For this review, take the finished solid that the model builds, in its own axes (mm). Face numbers are marked on the shaded views. A direction names the side the tool comes from. Round coordinates to 2 decimals unless told otherwise and drop trailing zeros. Loops run counter-clockwise (first coordinate to the right, second up) from the corner with the lowest first, then second, coordinate; pieces in that order, holes last.
1. Tool access review of the marked faces 1, 2 and 3: name each direction out of +Z, -Z, +X, -X, +Y, -Y from which nothing blocks a thin tool from reaching the whole face with its end or side.
2. Draft analysis for pull direction X (two halves, no side actions). For the marked faces 4, 5 and 6, state which applies: released by +X, released by -X, zero draft, split by the parting line, or undercut.
3. Clearance check with flat-ended pins moving along their axes: pin 1 Ø0.8 at (y, z) = (-4, 14.5) entering from -X (3 decimals); pin 2 Ø2 at (y, z) = (-2, 10) entering from +X (3 decimals); pin 3 Ø1.4 at (x, y) = (-7.5, -3.5) entering from -Z; pin 4 Ø4 at (x, y) = (-2.5, -3.5) entering from +Z. State where each tip first meets the part, or that it passes through.
4. Consider section A-A on z = 7.5. State the section outline as (x, y) points (3 decimals), then the cut area to 3 significant figures.
5. Consider section D-D on y = -2.5. State how many separate pieces and enclosed holes the cut face has, then the cut area to 3 significant figures.
6. To check wall thickness, follow line 1 along Y through (x, z) = (0, 8.5); line 2 along Z through (x, y) = (-6.5, -1.75); line 3 along Z through (x, y) = (3.5, -2.75). State the ranges of each line that lie inside material, in increasing order.
7. Consider section C-C on z = 11.25. State the section outline as (x, y) points (3 decimals).
from build123d import *

# Parameters (mm, degrees)
SKIZZE1_W                         = 6.675
SKIZZE1_H                         = 4.27
AUFSATZ_LINEAR_AUSTRAGEN1_DEPTH   = 10.4
SKIZZE1_3_W                       = 6.675
SKIZZE1_3_H                       = 1.68
AUFSATZ_LINEAR_AUSTRAGEN2_DEPTH   = 15.35
LINEAR_AUSTRAGEN_D_NN1_START      = 4.75
LINEAR_AUSTRAGEN_D_NN1_DEPTH      = 2
SKIZZE3_W                         = 0.5
SKIZZE3_H                         = 1.6
AUFSATZ_LINEAR_AUSTRAGEN3_DEPTH   = 4.8
SKIZZE4_W                         = 7.337223246
SKIZZE4_H                         = 4.95
SCHNITT_LINEAR_AUSTRAGEN1_DEPTH   = 8.85
AUFSATZ_LINEAR_AUSTRAGEN4_REACH   = 21.408
AUFSATZ_LINEAR_START              = 0.5
SKIZZE5_W                         = 5.4
SKIZZE5_H                         = 2
AUFSATZ_LINEAR_START_2            = -0.9
SKIZZE6_W                         = 0.55
SKIZZE6_H                         = 0.3
AUFSATZ_LINEAR_AUSTRAGEN5_DEPTH   = 3.5
AUFSATZ_LINEAR_AUSTRAGEN5_2_DEPTH = 3.5
SKIZZE6_3_W                       = 0.55
SKIZZE6_3_H                       = 0.2
AUFSATZ_LINEAR_AUSTRAGEN6_DEPTH   = 0.3
VERRUNDUNG1_R                     = 0.2
VERRUNDUNG2_R                     = 0.5
VERRUNDUNG3_R                     = 0.3
VERRUNDUNG4_R                     = 0.7
AUFSATZ_LINEAR_START_3            = -6.675
SKIZZE7_W                         = 2.54
SKIZZE7_H                         = 3.27
AUFSATZ_LINEAR_AUSTRAGEN7_DEPTH   = 0.25
VERRUNDUNG6_R                     = 0.5
VERRUNDUNG7_R                     = 0.5
LINEAR_AUSTRAGEN_D_NN2_DEPTH      = 0.7
VERRUNDUNG5_R                     = 0.7


with BuildPart() as part:
    # Skizze1 → Aufsatz-Linear austragen1 (new body)
    with BuildSketch(Plane.XY):
        with Locations((-3.3375, -3.815)):
            Rectangle(SKIZZE1_W, SKIZZE1_H)
    extrude(amount=AUFSATZ_LINEAR_AUSTRAGEN1_DEPTH)

    # Skizze1<3> → Aufsatz-Linear austragen2 (add)
    with BuildSketch(Plane.XY):
        with Locations((-3.3375, -0.84)):
            Rectangle(SKIZZE1_3_W, SKIZZE1_3_H)
    extrude(amount=AUFSATZ_LINEAR_AUSTRAGEN2_DEPTH)

    # Skizze2 → Linear-Austragen-Dünn1 (add)
    with BuildSketch(Plane.XY.offset(LINEAR_AUSTRAGEN_D_NN1_START)):
        with BuildLine():
            Line((0, -2.95), (-8.75, -2.95))
            ThreePointArc((-8.75, -2.95), (-9.13890873, -3.11109127), (-9.3, -3.5))
            Line((-9.3, -3.5), (-9.3, -4.7))
            Line((-9.3, -4.7), (-8.8, -4.7))
            Line((-8.8, -4.7), (-8.8, -3.5))
            ThreePointArc((-8.8, -3.5), (-8.785355339, -3.464644661), (-8.75, -3.45))
            Line((-8.75, -3.45), (0, -3.45))
            Line((0, -3.45), (0, -2.95))
        make_face()
    extrude(amount=LINEAR_AUSTRAGEN_D_NN1_DEPTH)

    # Skizze3 → Aufsatz-Linear austragen3 (add)
    with BuildSketch(Plane(origin=(0, 0, 0), x_dir=(1, 0, 0), z_dir=(0, 1, 0))):
        with Locations((-6.425, -14.55)):
            Rectangle(SKIZZE3_W, SKIZZE3_H)
    extrude(amount=-AUFSATZ_LINEAR_AUSTRAGEN3_DEPTH)

    # Skizze4 → Schnitt-Linear austragen1 (cut)
    with BuildSketch(Plane.XY):
        with Locations((-2.511388377, -2.975)):
            Rectangle(SKIZZE4_W, SKIZZE4_H)
    extrude(amount=SCHNITT_LINEAR_AUSTRAGEN1_DEPTH, mode=Mode.SUBTRACT)

    # Skizze5 → Aufsatz-Linear austragen4 (add, up to next)
    with BuildSketch(Plane.XY.offset(AUFSATZ_LINEAR_START), mode=Mode.PRIVATE) as aufsatz_linear_austragen4_sk1:
        with Locations((-2.7, -1.9)):
            Rectangle(SKIZZE5_W, SKIZZE5_H)
    aufsatz_linear_austragen4_tool1 = extrude(aufsatz_linear_austragen4_sk1.sketch, amount=AUFSATZ_LINEAR_AUSTRAGEN4_REACH, mode=Mode.PRIVATE) - part.part
    add(aufsatz_linear_austragen4_tool1.solids().sort_by_distance((-2.7, -1.9, 0.5))[0])



with BuildPart() as body_2:
    # Skizze6 → Aufsatz-Linear austragen5 (new body)
    with BuildSketch(Plane(origin=(0, 0, 0), x_dir=(1, 0, 0), z_dir=(0, 1, 0)).offset(AUFSATZ_LINEAR_START_2)):
        with Locations((-1, -15.7)):
            Rectangle(SKIZZE6_W, SKIZZE6_H)
    extrude(amount=-AUFSATZ_LINEAR_AUSTRAGEN5_DEPTH)


with BuildPart() as body_3:
    # Skizze6 → Aufsatz-Linear austragen5 2 (new body)
    with BuildSketch(Plane(origin=(0, 0, 0), x_dir=(1, 0, 0), z_dir=(0, 1, 0)).offset(AUFSATZ_LINEAR_START_2)):
        with Locations((-3.5, -15.7)):
            Rectangle(SKIZZE6_W, SKIZZE6_H)
    extrude(amount=-AUFSATZ_LINEAR_AUSTRAGEN5_2_DEPTH)


with BuildPart() as part_1:
    add(part.part)

    add(body_2.part)  # Aufsatz-Linear austragen6 merges body 2

    add(body_3.part)  # Aufsatz-Linear austragen6 merges body 3
    # Skizze6<3> → Aufsatz-Linear austragen6 (add)
    with BuildSketch(Plane(origin=(0, 0, 0), x_dir=(1, 0, 0), z_dir=(0, 1, 0)).offset(AUFSATZ_LINEAR_START_2)):
        with Locations((-3.5, -15.45)):
            Rectangle(SKIZZE6_3_W, SKIZZE6_3_H)
        with Locations((-1, -15.45)):
            Rectangle(SKIZZE6_3_W, SKIZZE6_3_H)
    extrude(amount=-AUFSATZ_LINEAR_AUSTRAGEN6_DEPTH)

    # Verrundung1
    verrundung1_edges = [part_1.edges().sort_by_distance(p)[0] for p in [
        (-3.5, -1.2, 15.55),
        (-1, -1.2, 15.55),
    ]]
    fillet(verrundung1_edges, radius=VERRUNDUNG1_R - 0.0001)  # a hair under: the kernel refuses the full size

    # Verrundung2
    verrundung2_edges = [part_1.edges().sort_by_distance(p)[0] for p in [
        (-1, -0.9, 15.85),
        (-3.5, -0.9, 15.85),
    ]]
    fillet(verrundung2_edges, radius=VERRUNDUNG2_R - 0.0001)  # a hair under: the kernel refuses the full size

    # Verrundung3
    verrundung3_edges = [part_1.edges().sort_by_distance(p)[0] for p in [
        (-6.18, -0.5, 4.425),
        (-6.18, -5.45, 4.425),
    ]]
    fillet(verrundung3_edges, radius=VERRUNDUNG3_R)

    # Verrundung4
    verrundung4_edges = [part_1.edges().sort_by_distance(p)[0] for p in [
        (-6.675, 0, 7.675),
        (-6.675, -5.95, 5.2),
    ]]
    fillet(verrundung4_edges, radius=VERRUNDUNG4_R)

    # Skizze7 → Aufsatz-Linear austragen7 (add)
    with BuildSketch(Plane(origin=(0, 0, 0), x_dir=(0, 0, -1), z_dir=(1, 0, 0)).offset(AUFSATZ_LINEAR_START_3)):
        with Locations((-9.13, -3.315)):
            Rectangle(SKIZZE7_W, SKIZZE7_H)
    extrude(amount=-AUFSATZ_LINEAR_AUSTRAGEN7_DEPTH)

    # Verrundung6
    verrundung6_edges = [part_1.edges().sort_by_distance(p)[0] for p in [
        (-9.05, -4.7, 4.75),
        (-9.05, -4.7, 6.75),
        (-6.425, -4.8, 13.75),
        (-6.425, -4.8, 15.35),
    ]]
    fillet(verrundung6_edges, radius=VERRUNDUNG6_R)

    # Verrundung7
    verrundung7_edges = [part_1.edges().sort_by_distance(p)[0] for p in [
        (-6.8, -1.68, 7.86),
        (-6.8, -4.95, 7.86),
    ]]
    fillet(verrundung7_edges, radius=VERRUNDUNG7_R)

    # Spiegeln1: part across plane


with BuildPart() as part_2:
    add(part_1.part)
    add(part_1.part.mirror(Plane(origin=(0, 0, 0), x_dir=(0, 0, 1), z_dir=(1, 0, 0))))

    # Skizze8 → Linear-Austragen-Dünn2 (add, symmetric)
    with BuildSketch(Plane(origin=(0, 0, 0), x_dir=(0, 0, -1), z_dir=(1, 0, 0))):
        with BuildLine():
            Line((-7.127333731, 0), (-9, 0))
            ThreePointArc((-9, 0), (-9.189684168, 0.027582553), (-9.363657097, 0.108045593))
            Line((-9.363657097, 0.108045593), (-13.2907964, 2.667554689))
            Line((-13.2907964, 2.667554689), (-13.5092036, 2.332445311))
            Line((-13.5092036, 2.332445311), (-9.582064297, -0.227063785))
            ThreePointArc((-9.582064297, -0.227063785), (-9.303605739, -0.355851764), (-9, -0.4))
            Line((-9, -0.4), (-7.127333731, -0.4))
            Line((-7.127333731, -0.4), (-7.127333731, 0))
        make_face()
    extrude(amount=LINEAR_AUSTRAGEN_D_NN2_DEPTH, both=True)

    # Verrundung5
    verrundung5_edges = [part_2.edges().sort_by_distance(p)[0] for p in [
        (-0.7, 2.5, 13.4),
        (0.7, 2.5, 13.4),
    ]]
    fillet(verrundung5_edges, radius=VERRUNDUNG5_R - 0.0001)  # a hair under: the kernel refuses the full size


solid = part_2.part
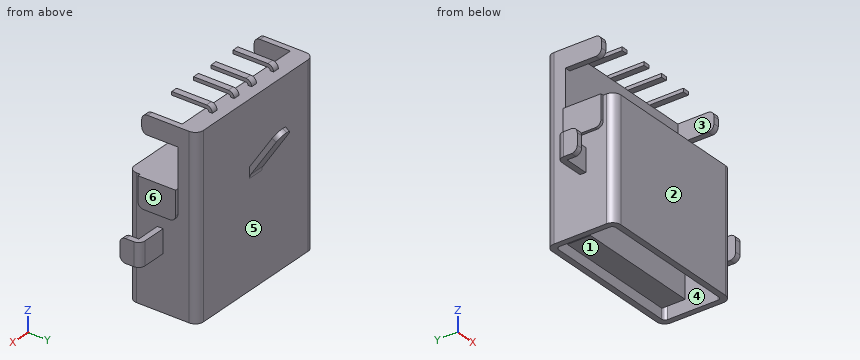
Resolved:
1. face 1: -Z
1. face 2: +Z, -Z, +X, -X, -Y
1. face 3: +Z, -Y
2. face 4: undercut
2. face 5: zero draft
2. face 6: released by +X
3. pin 1: stops at x = -6.675
3. pin 2: stops at x = 6.925
3. pin 3: stops at z = 4.75
3. pin 4: stops at z = 15.85
4. outline: (-6.675, -5.25) arc R0.7 ccw to (-5.975, -5.95) - (5.975, -5.95) arc R0.7 ccw to (6.675, -5.25) - (6.675, -0.7) arc R0.7 ccw to (5.975, 0) - (-5.975, 0) arc R0.7 ccw to (-6.675, -0.7) - close; (-5.4, -2.9) - (5.4, -2.9) - (5.4, -0.9) - (-5.4, -0.9) - close; hole (-6.18, -5.15) arc R0.3 ccw to (-5.88, -5.45) - (5.88, -5.45) arc R0.3 ccw to (6.18, -5.15) - (6.18, -0.8) arc R0.3 ccw to (5.88, -0.5) - (-5.88, -0.5) arc R0.3 ccw to (-6.18, -0.8) - close
4. area: 39.5 mm2
5. separate pieces: 7
5. enclosed holes: 0
5. area: 123 mm2
6. line 1: y = -5.95 to -5.45, -2.9 to -0.9, -0.5 to 0
6. line 2: z = 0 to 10.4, 13.75 to 15.35
6. line 3: z = 0.5 to 10.4, 15.55 to 15.85
7. outline: (-6.675, -1.68) - (6.675, -1.68) - (6.675, -0.7) arc R0.7 ccw to (5.975, 0) - (-5.975, 0) arc R0.7 ccw to (-6.675, -0.7) - close; (-0.7, 0.86) - (0.7, 0.86) - (0.7, 1.337) - (-0.7, 1.337) - close
